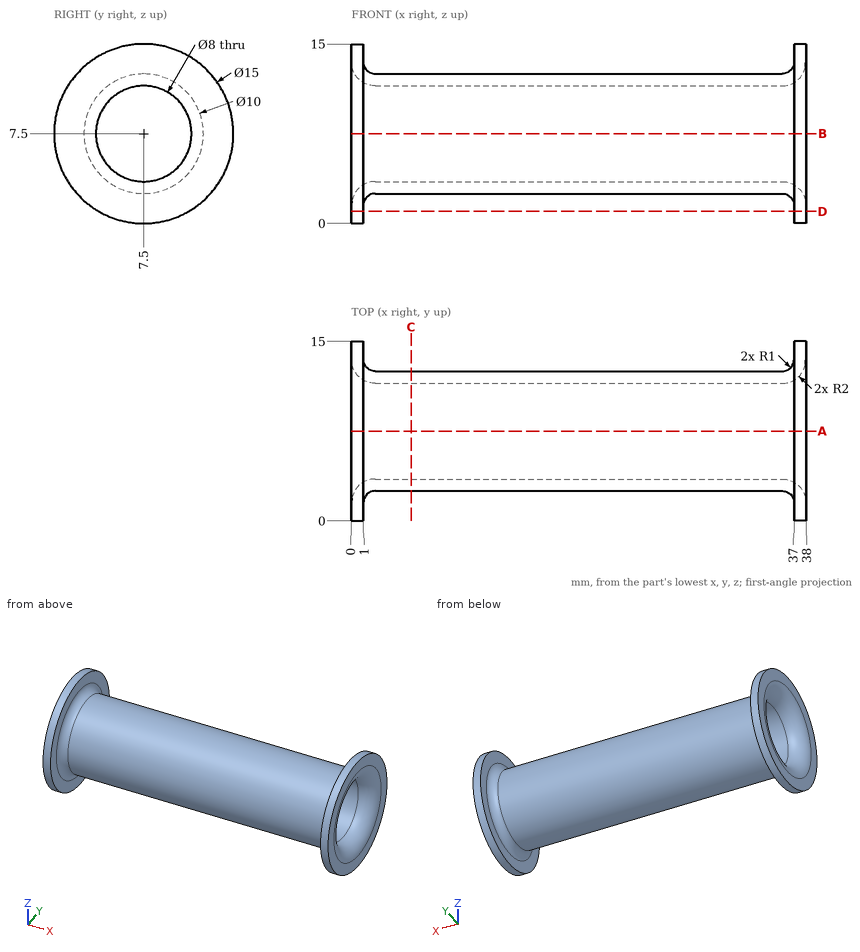
Design review of the part shown in the three views and the two pictorial views. Dimensions are in mm from the part's minimum x, y and z. Give positions to 0.01 mm unless a question says otherwise; leave off trailing zeros. Loops run counter-clockwise (first coordinate to the right, second up) from the corner with the lowest first, then second, coordinate; pieces in that order, holes last. Notation, with made-up numbers: M 43,19.25 L 80,19.25 A19 ccw 80,24.25 Z; hole C 73,-3 d4. An arc over 180 degrees is marked long. Answer as a JSON object with one key per item and string values. Group by question number.
Q1. Insertion check: P1, Ø2, axis at y = 10, z = 10, coming from the -X side; P2, Ø1, axis at x = 20, y = 10.5, coming from the -Z side; P3, Ø6, axis at x = 14.5, z = 6.5, coming from the -Y side. Each pin has a flat end and moves straight along its axis. Give the tip position at first contact, or say it passes through.
Q2. Add section C-C on x = 5. Give the boundary of the cut face in (y, z).
Q3. Add section D-D on z = 1. Give the boundary of the cut face in (x, y).
Q4. For probe 1 along X at (y, z) = (8.25, 14.5); probe 2 along Y at (x, z) = (12.5, 7.5); probe 3 along Z at (x, y) = (30, 10.5), list the stretches that pass through material, from the lowest coordinate up. Write a range as [from, to].
Q5. Add section A-A on y = 7.5. Give the boundary of the cut face in (x, z).
Checked values:
{
 "1": {"P1": "x = 0.64", "P2": "z = 3.17", "P3": "y = 2.5"},
 "2": {"outline": "C 7.5,7.5 d10; hole C 7.5,7.5 d8"},
 "3": {"outline": "M 0,3.76 L 1,3.76 L 1,11.24 L 0,11.24 Z; M 37,3.76 L 38,3.76 L 38,11.24 L 37,11.24 Z"},
 "4": {"probe 1": "[0, 1], [37, 38]", "probe 2": "[2.5, 3.5], [11.5, 12.5]", "probe 3": "[3.5, 4.85], [10.15, 11.5]"},
 "5": {"outline": "M 0,0 L 1,0 L 1,1.5 A1 cw 2,2.5 L 36,2.5 A1 cw 37,1.5 L 37,0 L 38,0 L 38,1.5 A2 ccw 36,3.5 L 2,3.5 A2 ccw 0,1.5 Z; M 0,13.5 A2 ccw 2,11.5 L 36,11.5 A2 ccw 38,13.5 L 38,15 L 37,15 L 37,13.5 A1 cw 36,12.5 L 2,12.5 A1 cw 1,13.5 L 1,15 L 0,15 Z"}
}
